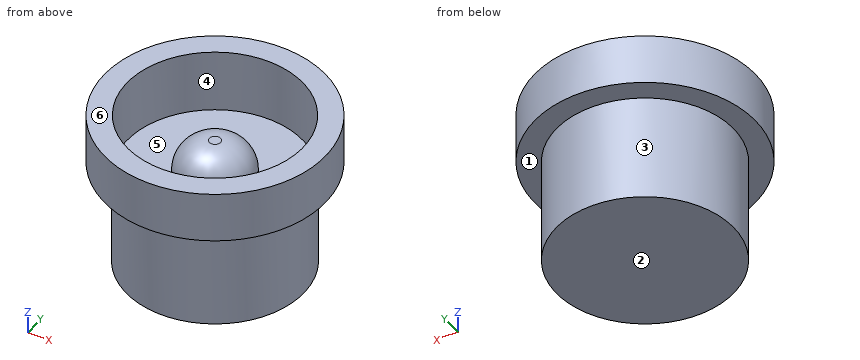
```python
from build123d import *

# Parameters (mm, degrees)
F2_R     = 8.5041977155
F3_DEPTH = 6.0452
F4_R     = 3.5986110649
F5_DEPTH = 3.4036
F6_R     = 3.048


# Not quite as in the source:
# - a feature of the source that left no trace in its solid (it failed there, or was rolled back) is left out


with BuildPart() as f1:
    # F0 (on Front) → F1 (revolve)
    with BuildSketch(Plane.XZ):
        Polygon((0, -7.3331215731), (0, 7.9068784269), (-10.6934, 7.9068784269), (-10.6934, 3.0300784269), (-8.5852, 3.0300784269), (-8.5852, -7.3331215731), align=None)
    revolve(axis=Axis((0, 0, 0.2868784269), (0, 0, 1)))

    # F2 (on face) → F3 (cut)
    with BuildSketch(Plane.XY.offset(7.9068784269)):
        Circle(F2_R)
    extrude(amount=-F3_DEPTH, mode=Mode.SUBTRACT)

    # F4 (on face) → F5 (join)
    with BuildSketch(Plane.XY.offset(1.8616784269)):
        Circle(F4_R)
    extrude(amount=F5_DEPTH)

    # F6
    f6_edges = [f1.edges().sort_by_distance(p)[0] for p in [
        (-3.598611, 0, 5.265278),
    ]]
    fillet(f6_edges, radius=F6_R)


solid = f1.part
```
Geometry check sheet. Reference: the model listing, model coordinates, mm. Face numbers are marked on the shaded views. A direction names the side the tool comes from. Give positions to 0.01 mm unless a question says otherwise; leave off trailing zeros. Order: outer loops, then holes, each group sorted by start corner. A loop starts at its lowest first (then second) coordinate and runs counter-clockwise, first axis right, second up.
1. Release check for a two-part mould opening along X. For the marked faces 3, 4, 5 and 6 record: pulls with the +X half, pulls with the -X half, needs draft (parallel to the pull), parting line crosses it, or undercut.
2. Gauge pin test, flat ends, axial feed: pin 1 Ø1 at (y, z) = (8, 5.5) entering from -X; pin 2 Ø2 at (y, z) = (-5, 0) entering from +X; pin 3 Ø4 at (x, z) = (-2.5, 0.5) entering from +Y. Record the tip position at first contact, or that the pin passes through.
3. Section check B-B, the plane x = -7.25. Enter the section's corners in (y, z).
4. Access from +Z, -Z, +X, -X, +Y, -Y to the whole of each face (thin tool, end or side, straight path). Record for the marked faces 1 and 2.
5. Section check C-C, the plane z = -2.75. Enter the section's corners in (x, y), and give its area (3 significant figures).
6. Thickness scan on L1, parallel to Y at x = 0, z = 4.75; L2, parallel to Y at x = 0, z = 3.5; L3, parallel to Y at x = 0, z = 5.75. Record the ranges inside material, lowest first.
7. Section check A-A, the plane y = 4. Enter the section's corners in (x, z).
Values follow:
1. face 3: parting line crosses it
1. face 4: undercut
1. face 5: undercut
1. face 6: needs draft
2. pin 1: stops at x = -7.62
2. pin 2: stops at x = 7.6
2. pin 3: stops at y = 8.57
3. outline: (-7.86, 3.03) - (-4.6, 3.03) - (-4.6, -7.33) - (4.6, -7.33) - (4.6, 3.03) - (7.86, 3.03) - (7.86, 7.91) - (4.45, 7.91) - (4.45, 1.86) - (-4.45, 1.86) - (-4.45, 7.91) - (-7.86, 7.91) - close
4. face 1: -Z
4. face 2: -Z, +X, -X, +Y, -Y
5. outline: circle Ø17.17 at (0, 0)
5. area: 232 mm2
6. L1: y = -10.69 to -8.5, -2.25 to 2.25, 8.5 to 10.69
6. L2: y = -10.69 to -8.5, -3.32 to 3.32, 8.5 to 10.69
6. L3: y = -10.69 to -8.5, 8.5 to 10.69
7. outline: (-9.92, 3.03) - (-7.6, 3.03) - (-7.6, -7.33) - (7.6, -7.33) - (7.6, 3.03) - (9.92, 3.03) - (9.92, 7.91) - (7.5, 7.91) - (7.5, 1.86) - (-7.5, 1.86) - (-7.5, 7.91) - (-9.92, 7.91) - close
